CAD build for the part. Positions are in the model's coordinates, mm. Round coordinates to 2 decimals unless told otherwise and drop trailing zeros. Write each loop counter-clockwise with the first axis right and the second up, starting at its lowest first coordinate (ties: lowest second). Pieces come first, ordered by that corner, then holes. Notation, with made-up numbers: M 36.5,79 L 52.5,79 A24 ccw 52.5,110 Z; hole C 52.25,10 d6. An arc over 180 degrees is marked long. Write each question's results on one line, items separated by ' | '. Start each with the question number.
```python
from build123d import *

# Parameters (mm, degrees)
SKETCH1_W           = 42
SKETCH1_H           = 100
BOSS_EXTRUDE1_DEPTH = 2
SKETCH2_R           = 1.5
CUT_EXTRUDE1_DEPTH  = 2


with BuildPart() as part:
    # Sketch1 → Boss-Extrude1 (new body)
    with BuildSketch(Plane.XY):
        Rectangle(SKETCH1_W, SKETCH1_H)
    extrude(amount=BOSS_EXTRUDE1_DEPTH)

    # Sketch2 → Cut-Extrude1 (cut)
    with BuildSketch(Plane.XY.offset(2)):
        with Locations((-13, -40)):
            Circle(SKETCH2_R)
        with Locations((13, -40)):
            Circle(SKETCH2_R)
        with Locations(Location((13, -14, 0), (0, 0, 180))):
            Circle(SKETCH2_R)
        with Locations(Location((-13, -14, 0), (0, 0, 180))):
            Circle(SKETCH2_R)
        with Locations(Location((13, 40, 0), (0, 0, 180))):
            Circle(SKETCH2_R)
        with Locations(Location((-13, 40, 0), (0, 0, 180))):
            Circle(SKETCH2_R)
        with Locations((13, 14)):
            Circle(SKETCH2_R)
        with Locations((-13, 14)):
            Circle(SKETCH2_R)
    extrude(amount=-CUT_EXTRUDE1_DEPTH, mode=Mode.SUBTRACT)


solid = part.part
```
1) Saw through at A-A, the plane y = 14. Write the cut outline in (x, z), plus the area to 3 significant figures.
2) Saw through at B-B, the plane x = -13. Write the cut outline in (y, z), plus the area to 3 significant figures.
3) Pull direction X, two halves, no side cores. Call faces 1 (the face through (-14.5, 14.07, 1.01)), 2 (the face through (21, -1, 1)), 3 (the face through (0, 50, 1)): pulls with the +X half, pulls with the -X half, needs draft (parallel to the pull), parting line crosses it, or undercut.
4) Wall check: line 1 along X through (y, z) = (-14, 1.25); line 2 along Y through (x, z) = (13, 1.4). Give the ranges that are in metal, low to high. Write a range as from..to.
Filled sheet:
1) outline: M -21,0 L -14.5,0 L -14.5,2 L -21,2 Z; M -11.5,0 L 11.5,0 L 11.5,2 L -11.5,2 Z; M 14.5,0 L 21,0 L 21,2 L 14.5,2 Z | area: 72.0 mm^2
2) outline: M -50,0 L -41.5,0 L -41.5,2 L -50,2 Z; M -38.5,0 L -15.5,0 L -15.5,2 L -38.5,2 Z; M -12.5,0 L 12.5,0 L 12.5,2 L -12.5,2 Z; M 15.5,0 L 38.5,0 L 38.5,2 L 15.5,2 Z; M 41.5,0 L 50,0 L 50,2 L 41.5,2 Z | area: 176 mm^2
3) face 1: undercut | face 2: pulls with the +X half | face 3: needs draft
4) line 1: x = -21..-14.5, -11.5..11.5, 14.5..21 | line 2: y = -50..-41.5, -38.5..-15.5, -12.5..12.5, 15.5..38.5, 41.5..50
